Part model, mm, in its own coordinate system. Coordinates: 2 decimals unless noted, no trailing zeros. Loops run counter-clockwise (first coordinate to the right, second up) from the corner with the lowest first, then second, coordinate; pieces in that order, holes last. Notation, with made-up numbers: (69, -18) - (121, -18) arc R21 ccw to (121, -1) - close; hole circle Ø10 at (-18.5, -13.75). An arc over 180 degrees is marked (long way). Use a Markdown table: item, result. Add a question column.
1. Wall check: probe 1 along Y at (x, z) = (0, 0.7) (3 decimals); probe 2 along X at (y, z) = (32, 0.3); probe 3 along Y at (x, z) = (124, 0.85). Give the ranges that are in metal, low to high. Write a range as [from, to].
2. Band-saw the part on D-D, the plane x = 68.5. Give the cut face in (y, z), plus the area to 3 significant figures.
3. Band-saw the part on B-B, the plane z = 0.4. Give the cut face in (x, y) (3 decimals).
4. Band-saw the part on C-C, the plane y = 0. Give the cut face in (x, z) (3 decimals), plus the area to 3 significant figures.
5. Band-saw the part on A-A, the plane x = 0. Give the cut face in (y, z) (3 decimals).
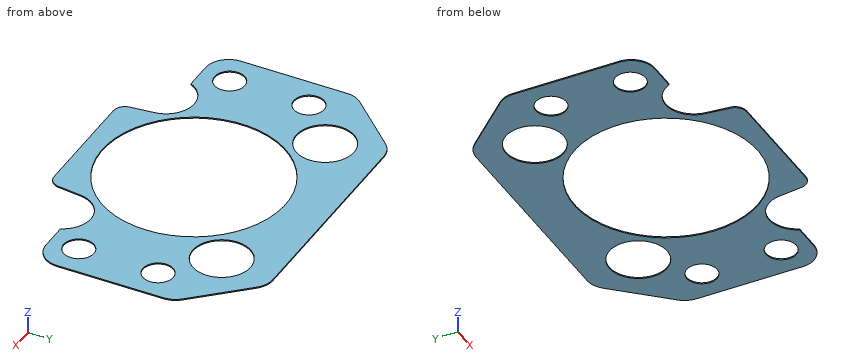
from build123d import *

# Parameters (mm, degrees)
SKETCH1_R           = 24.75
SKETCH1_R_2         = 13
SKETCH1_R_3         = 78.475
BOSS_EXTRUDE1_DEPTH = 1


with BuildPart() as part:
    # Sketch1 → Boss-Extrude1 (new body)
    with BuildSketch(Plane.XY):
        with BuildLine():
            Line((-2.561737691, 115.5), (-91.270303138, 115.5))
            ThreePointArc((-91.270303138, 115.5), (-99.271058557, 113.829973069), (-105.935666275, 109.098791272))
            Line((-105.935666275, 109.098791272), (-145.665363137, 66.253039754))
            ThreePointArc((-145.665363137, 66.253039754), (-149.618636668, 59.958108327), (-151, 52.654248482))
            Line((-151, 52.654248482), (-151, -38.5))
            ThreePointArc((-151, -38.5), (-145.142135624, -52.642135624), (-131, -58.5))
            Line((-131, -58.5), (-107.203603311, -58.5))
            ThreePointArc((-107.203603311, -58.5), (-81.413958175, -44.266614), (-60.915571747, -65.421075164))
            Line((-60.915571747, -65.421075164), (-58.537563271, -85.666566943))
            ThreePointArc((-58.537563271, -85.666566943), (-55.251678473, -91.972137225), (-48.60584028, -94.5))
            Line((-48.60584028, -94.5), (48.60584028, -94.5))
            ThreePointArc((48.60584028, -94.5), (55.251678473, -91.972137225), (58.537563271, -85.666566943))
            Line((58.537563271, -85.666566943), (60.915571747, -65.421075164))
            ThreePointArc((60.915571747, -65.421075164), (81.413958175, -44.266614), (107.203603311, -58.5))
            Line((107.203603311, -58.5), (131, -58.5))
            ThreePointArc((131, -58.5), (145.142135624, -52.642135624), (151, -38.5))
            Line((151, -38.5), (151, 52.654248482))
            ThreePointArc((151, 52.654248482), (149.618636668, 59.958108327), (145.665363137, 66.253039754))
            Line((145.665363137, 66.253039754), (105.935666275, 109.098791272))
            ThreePointArc((105.935666275, 109.098791272), (99.271058557, 113.829973069), (91.270303138, 115.5))
            Line((91.270303138, 115.5), (-2.561737691, 115.5))
        make_face()
        with Locations((-85, 68.25)):
            Circle(SKETCH1_R, mode=Mode.SUBTRACT)
        with Locations((85, 68.25)):
            Circle(SKETCH1_R, mode=Mode.SUBTRACT)
        with Locations((124, -34)):
            Circle(SKETCH1_R_2, mode=Mode.SUBTRACT)
        with Locations((124, 34)):
            Circle(SKETCH1_R_2, mode=Mode.SUBTRACT)
        with Locations((-124, 34)):
            Circle(SKETCH1_R_2, mode=Mode.SUBTRACT)
        with Locations((-124, -34)):
            Circle(SKETCH1_R_2, mode=Mode.SUBTRACT)
        Circle(SKETCH1_R_3, mode=Mode.SUBTRACT)
    extrude(amount=BOSS_EXTRUDE1_DEPTH)


solid = part.part
Geometry check:
| question | item | result |
|---|---|---|
| 1 | probe 1 | y = [-94.5, -78.475], [78.475, 115.5] |
| 1 | probe 2 | x = [-151, -136.85], [-111.15, -71.65], [71.65, 111.15], [136.85, 151] |
| 1 | probe 3 | y = [-58.5, -47], [-21, 21], [47, 89.62] |
| 2 | outline | (-50.48, 0) - (-38.29, 0) - (-38.29, 1) - (-50.48, 1) - close; (38.29, 0) - (49.8, 0) - (49.8, 1) - (38.29, 1) - close; (86.7, 0) - (115.5, 0) - (115.5, 1) - (86.7, 1) - close |
| 2 | area | 52.5 mm^2 |
| 3 | outline | (-151, -38.5) arc R20 ccw to (-131, -58.5) - (-107.204, -58.5) arc R24.25 cw to (-60.916, -65.421) - (-58.538, -85.667) arc R10 ccw to (-48.606, -94.5) - (48.606, -94.5) arc R10 ccw to (58.538, -85.667) - (60.916, -65.421) arc R24.25 cw to (107.204, -58.5) - (131, -58.5) arc R20 ccw to (151, -38.5) - (151, 52.654) arc R20 ccw to (145.665, 66.253) - (105.936, 109.099) arc R20 ccw to (91.27, 115.5) - (-91.27, 115.5) arc R20 ccw to (-105.936, 109.099) - (-145.665, 66.253) arc R20 ccw to (-151, 52.654) - close; hole circle Ø26 at (-124, -34); hole circle Ø26 at (-124, 34); hole circle Ø49.5 at (-85, 68.25); hole circle Ø156.95 at (0, 0); hole circle Ø49.5 at (85, 68.25); hole circle Ø26 at (124, -34); hole circle Ø26 at (124, 34) |
| 4 | outline | (-151, 0) - (-78.475, 0) - (-78.475, 1) - (-151, 1) - close; (78.475, 0) - (151, 0) - (151, 1) - (78.475, 1) - close |
| 4 | area | 145 mm^2 |
| 5 | outline | (-94.5, 0) - (-78.475, 0) - (-78.475, 1) - (-94.5, 1) - close; (78.475, 0) - (115.5, 0) - (115.5, 1) - (78.475, 1) - close |
